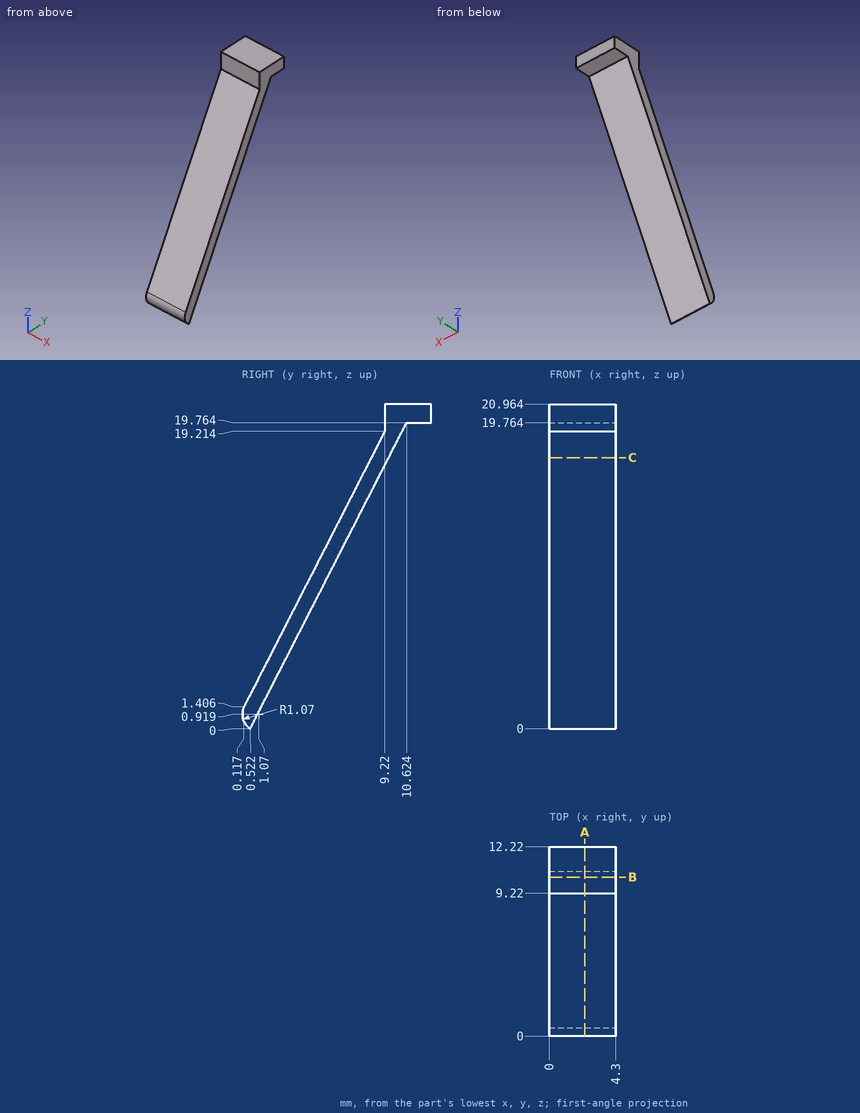
The drawing under review shows one solid part. Ordinate dimensions are in mm from its lowest x, y, z. Round coordinates to 2 decimals unless told otherwise and drop trailing zeros. Loops run counter-clockwise (first coordinate to the right, second up) from the corner with the lowest first, then second, coordinate; pieces in that order, holes last. Notation, with made-up numbers: (68, -38.75) - (113, -38.75) arc R21 cw to (113, -13.75) - close; hole circle Ø2 at (-8.75, -13). An arc over 180 degrees is marked (long way). One line per question, with ' | ' between items.
Q1. Take a section at B-B (y = 10.25). Give the boundary of the cut face in (x, z).
Taken from the geometry:
outline: (0, 19.03) - (4.3, 19.03) - (4.3, 20.96) - (0, 20.96) - close
Q2. For line 1 along Z through (x, y) = (1.8, 10.75); line 2 along Y through (x, z) = (3.2, 19.5); line 3 along Y through (x, z) = (0.9, 4), list the stretches that pass through material, from the lowest coordinate up. Write a range as [from, to].
Taken from the geometry:
line 1: z = [19.76, 20.96] | line 2: y = [9.22, 10.49] | line 3: y = [1.44, 2.57]
Q3. Take a section at C-C (z = 17.5). Give the boundary of the cut face in (x, y).
Taken from the geometry:
outline: (0, 8.34) - (4.3, 8.34) - (4.3, 9.47) - (0, 9.47) - close
Q4. Take a section at A-A (x = 2.3). Give the boundary of the cut face in (y, z).
Taken from the geometry:
outline: (0.12, 1.41) arc R1.07 ccw to (0.52, 0) - (10.62, 19.76) - (12.22, 19.76) - (12.22, 20.96) - (9.22, 20.96) - (9.22, 19.21) - close
Q5. For pin 1 (0.9 mm diameter, centred on x = 2.5, z = 19.5, fed in from -Y) (1 decimal); pin 2 (2 mm diameter, centred on x = 1, z = 11.5, fed in from +Y); pin 3 (1 mm diameter, centred on x = 3, y = 7.5, fed in from +Z), all flat-tipped, find the tip position at first contact; note any pin that passes through.
Taken from the geometry:
pin 1: stops at y = 9.1 | pin 2: stops at y = 6.91 | pin 3: stops at z = 16.83
